```python
from build123d import *

# Parameters (mm, degrees)
F1_DEPTH = 76.2
F2_R     = 19.05
F3_DEPTH = 12.7
F4_DEPTH = 76.2
F5_R     = 12.7
F6_DEPTH = 25374.6


with BuildPart() as f1:
    # F0 (on Front) → F1 (new body)
    with BuildSketch(Plane.XZ):
        Polygon((0, 155.575), (0, 0), (177.8, 0), (177.8, 28.575), (82.55, 28.575), (82.55, 155.575), align=None)
    extrude(amount=F1_DEPTH)

    # F2 (on face) → F3 (cut)
    with BuildSketch(Plane.XZ.offset(76.2)):
        with Locations((41.275, 76.2)):
            Circle(F2_R)
    extrude(amount=-F3_DEPTH, mode=Mode.SUBTRACT)

    # F2 (on face) → F4 (cut)
    with BuildSketch(Plane.XZ.offset(76.2)):
        with BuildLine():
            Line((0, 155.575), (0, 76.2))
            ThreePointArc((0, 76.2), (41.275, 117.475), (82.55, 76.2))
            Line((82.55, 76.2), (82.55, 155.575))
            Line((82.55, 155.575), (0, 155.575))
        make_face()
    extrude(amount=-F4_DEPTH, mode=Mode.SUBTRACT)

    # F5 (on face) → F6 (cut)
    with BuildSketch(Plane.XY.offset(28.575)):
        with Locations((139.7, -38.1)):
            Circle(F5_R)
    extrude(amount=-F6_DEPTH, mode=Mode.SUBTRACT)


solid = f1.part
```
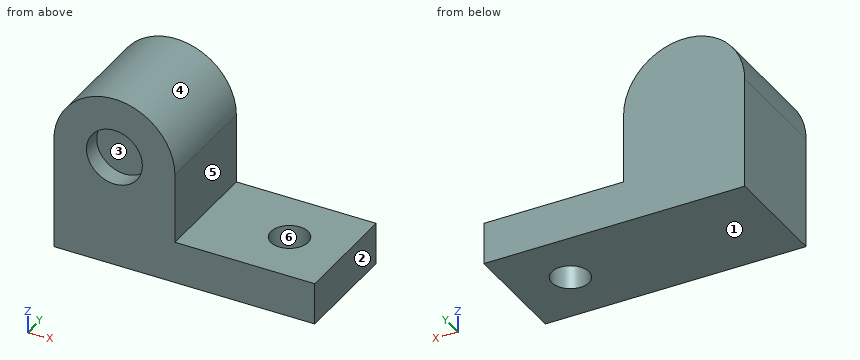
Geometry check sheet. Reference: the model listing, model coordinates, mm. Face numbers are marked on the shaded views. A direction names the side the tool comes from. Coordinates: 2 decimals unless noted, no trailing zeros. Write each loop counter-clockwise with the first axis right and the second up, starting at its lowest first coordinate (ties: lowest second). Pieces come first, ordered by that corner, then holes. Notation, with made-up numbers: (4.25, 86) -> (42.25, 86) arc R23 cw to (42.25, 113) -> close; hole circle Ø9 at (-1, -17.75). An arc over 180 degrees is marked (long way). Use CSV: the item, a comma, the result in double quotes. Start each with the question number.
Item 1: Cross-section at D-D, the plane z = 24. Record the cut outline in (x, y).
Item 2: Set-up check for the marked faces 5 and 6: record each of +Z, -Z, +X, -X, +Y, -Y from which the full face is reachable in a straight line by a thin tool's end or side.
Item 3: Mould release check, pull along Z, two halves, no side actions. Record for the marked faces 1, 2, 3 and 4: released by +Z, released by -Z, zero draft, split by the parting line, or undercut.
Item 4: Cross-section at A-A, the plane y = -38.1. Record the cut outline in (x, z) (3 decimals), plus the area to 3 significant figures.
Item 5: Cross-section at B-B, the plane x = 139.7. Record the cut outline in (y, z) (3 decimals).
Item 6: Depth check by flat-ended pin: pin 1 Ø14.5 at (y, z) = (-50.5, 49.5) entering from +X; pin 2 Ø1.5 at (x, y) = (93, -41.5) entering from +Z (3 decimals); pin 3 Ø15 at (x, y) = (139.7, -38.1) entering from +Z; pin 4 Ø12 at (x, y) = (28.5, -30.5) entering from +Z. Enter the tip coordinate at first touch or a pass-through.
Item 7: Thickness scan on line 1 (X direction, y = -71, z = 76); line 2 (X direction, y = -38, z = 19); line 3 (Z direction, x = 142, y = -4.5) (3 decimals). Record the ranges inside material, lowest first.
Item 8: Cross-section at C-C, the plane y = -69. Record the cut outline in (x, z) (3 decimals), plus the area to 3 significant figures.
Answers:
1,outline,"(0, -76.2) -> (177.8, -76.2) -> (177.8, 0) -> (0, 0) -> close; hole circle Ø25.4 at (139.7, -38.1)"
2,face 5,"+Z, +X, +Y, -Y"
2,face 6,"+Z, -Z"
3,face 1,"released by -Z"
3,face 2,"zero draft"
3,face 3,"undercut"
3,face 4,"released by +Z"
4,outline,"(0, 0) -> (127, 0) -> (127, 28.575) -> (82.55, 28.575) -> (82.55, 76.2) arc R41.275 ccw to (0, 76.2) -> close; (152.4, 0) -> (177.8, 0) -> (177.8, 28.575) -> (152.4, 28.575) -> close"
4,area,"11,000 mm^2"
5,outline,"(-76.2, 0) -> (-50.8, 0) -> (-50.8, 28.575) -> (-76.2, 28.575) -> close; (-25.4, 0) -> (0, 0) -> (0, 28.575) -> (-25.4, 28.575) -> close"
6,pin 1,"x = 82.55"
6,pin 2,"z = 28.575"
6,pin 3,"through"
6,pin 4,"z = 116.92"
7,line 1,"0 to 22.23, 60.32 to 82.55"
7,line 2,"0 to 127, 152.4 to 177.8"
7,line 3,"0 to 28.575"
8,outline,"(0, 0) -> (177.8, 0) -> (177.8, 28.575) -> (82.55, 28.575) -> (82.55, 76.2) arc R41.275 ccw to (0, 76.2) -> close; hole circle Ø38.1 at (41.275, 76.2)"
8,area,"10,500 mm^2"
